Geometry check sheet. Reference: drawing and pictorial views, mm from the part's lowest x, y, z. Give positions to 0.01 mm unless a question says otherwise; leave off trailing zeros. Order: outer loops, then holes, each group sorted by start corner. A loop starts at its lowest first (then second) coordinate and runs counter-clockwise, first axis right, second up.
Item 1: Sectioned sample at C-C on z = 82. Record the boundary of the cut face in (x, y), and give its area (3 significant figures).
Item 2: Sectioned sample at D-D on y = 57.5. Record the boundary of the cut face in (x, z), and give its area (3 significant figures).
Item 3: Release check for a two-part mould opening along Z. For the marked faces 1, 2 and 3 record: released by +Z, released by -Z, zero draft, split by the parting line, or undercut.
Item 4: Sectioned sample at B-B on x = 25.5. Record the boundary of the cut face in (y, z).
Item 5: Gauge pin test, flat ends, axial feed: P1, Ø2, axis at x = 46.5, y = 13.5, coming from the -Z side; P2, Ø4, axis at x = 32.5, z = 55, coming from the +Y side. Record the tip position at first contact, or that the pin passes through.
Item 6: Sectioned sample at A-A on y = 17. Record the boundary of the cut face in (x, z).
Item 7: Material ranges on line 1 along Z through (x, y) = (32.5, 47); line 2 along X through (y, z) = (58, 55); line 3 along Z through (x, y) = (32.5, 55.5), recorded low to high.
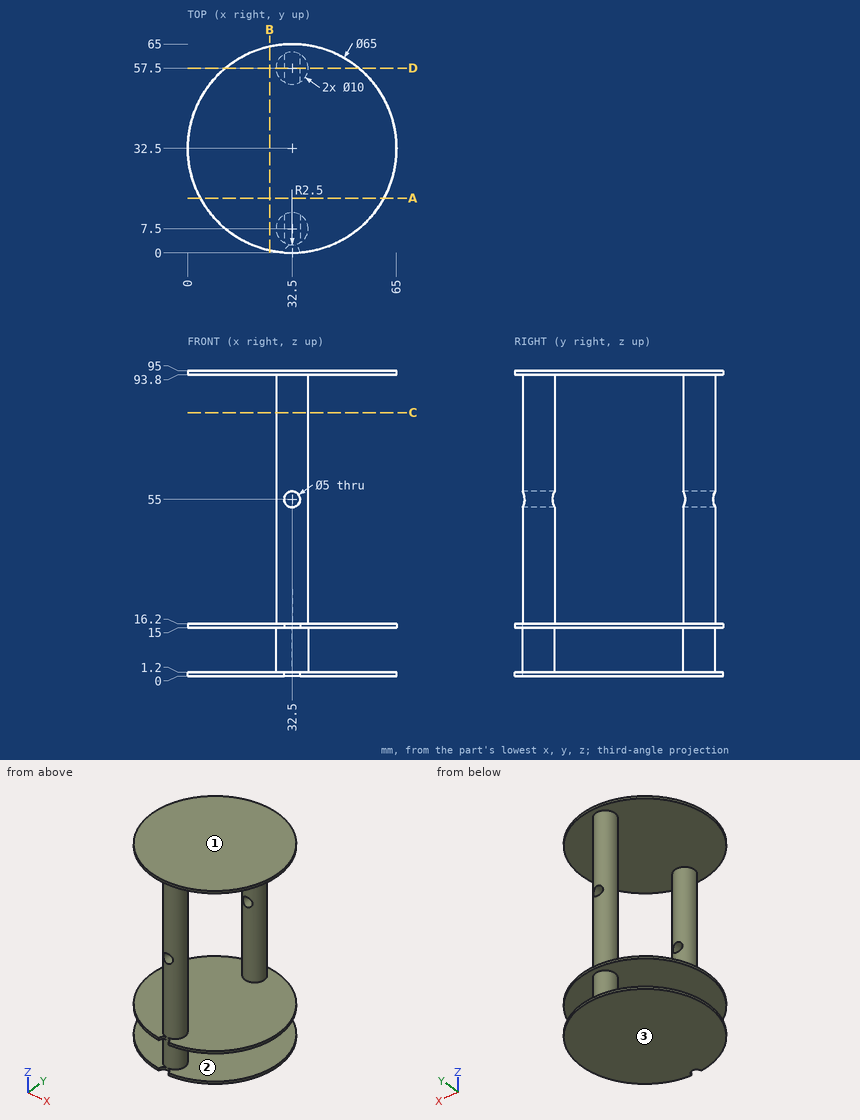
Report:
1. outline: circle Ø10 at (32.5, 7.5); circle Ø10 at (32.5, 57.5)
1. area: 157 mm2
2. outline: (11.73, 0) - (53.27, 0) - (53.27, 1.2) - (37.5, 1.2) - (37.5, 15) - (53.27, 15) - (53.27, 16.2) - (37.5, 16.2) - (37.5, 93.8) - (53.27, 93.8) - (53.27, 95) - (11.73, 95) - (11.73, 93.8) - (27.5, 93.8) - (27.5, 16.2) - (11.73, 16.2) - (11.73, 15) - (27.5, 15) - (27.5, 1.2) - (11.73, 1.2) - close; hole circle Ø5 at (32.5, 55)
2. area: 1,040 mm2
3. face 1: released by +Z
3. face 2: undercut
3. face 3: released by -Z
4. outline: (0.76, 0) - (64.24, 0) - (64.24, 1.2) - (0.76, 1.2) - close; (0.76, 15) - (64.24, 15) - (64.24, 16.2) - (0.76, 16.2) - close; (0.76, 93.8) - (64.24, 93.8) - (64.24, 95) - (0.76, 95) - close
5. P1: stops at z = 0
5. P2: passes through
6. outline: (3.93, 0) - (61.07, 0) - (61.07, 1.2) - (3.93, 1.2) - close; (3.93, 15) - (61.07, 15) - (61.07, 16.2) - (3.93, 16.2) - close; (3.93, 93.8) - (61.07, 93.8) - (61.07, 95) - (3.93, 95) - close
7. line 1: z = 0 to 1.2, 15 to 16.2, 93.8 to 95
7. line 2: x = 27.53 to 30, 35 to 37.47
7. line 3: z = 0 to 52.5, 57.5 to 95
